Job drawing, mm, ordinate dimensions from the low corner. One solid piece. Round coordinates to 2 decimals unless told otherwise and drop trailing zeros. Order: outer loops, then holes, each group sorted by start corner. A loop starts at its lowest first (then second) coordinate and runs counter-clockwise, first axis right, second up. Notation, with made-up numbers: (86, -30.5) -> (100, -30.5) arc R12 ccw to (100, -15.5) -> close; hole circle Ø3 at (74.25, -16.75). An arc over 180 degrees is marked (long way). Write item = value, one per line.
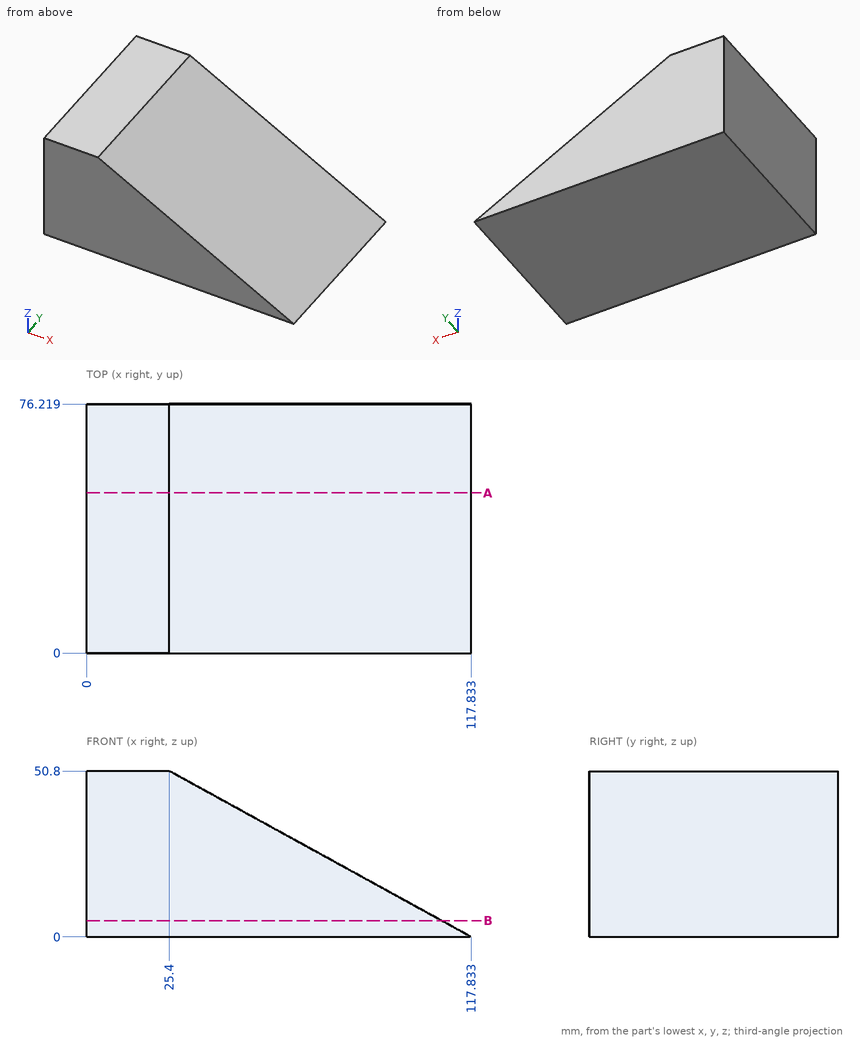
Q1. Cut at B-B, the plane z = 5. List the corners of the cut face in (x, y) (1 decimal).
Check values:
outline = (0, 0) -> (108.7, 0) -> (108.7, 76.2) -> (0, 76.2) -> close
Q2. Cut at A-A, the plane y = 49. List the corners of the cut face in (x, z).
Check values:
outline = (0, 0) -> (117.83, 0) -> (25.4, 50.8) -> (0, 50.8) -> close
Q3. Flat gauge pins, fed straight in: pin 1 (3 mm diameter, centred on y = 64.5, z = 8.5, fed in from +X) (1 decimal); pin 2 (2 mm diameter, centred on y = 50.5, z = 36.5, fed in from +X); pin 3 (10 mm diameter, centred on x = 48, y = 9, fed in from +Z). Where does each tip first touch, or does it go through?
Check values:
pin_1 = 105.1
pin_2 = 53.24
pin_3 = 41.13
Q4. Probe probe 1 along X at (y, z) = (61.5, 20.5) (1 decimal); probe 2 along X at (y, z) = (55.5, 3) (1 decimal); probe 3 along Z at (x, y) = (40, 72) (1 decimal). List the from-to ranges inside material, lowest first.
Check values:
probe_1 = 0 to 80.5
probe_2 = 0 to 112.4
probe_3 = 0 to 42.8
